from build123d import *

# Parameters (mm, degrees)
F0_W     = 44
F0_H     = 69
F1_DEPTH = 1200
F2_W     = 20
F2_H     = 44
F3_DEPTH = 44.001


with BuildPart() as f1:
    # F0 (on Top) → F1 (new body)
    with BuildSketch(Plane.XY):
        Rectangle(F0_W, F0_H)
    extrude(amount=F1_DEPTH)

    # F2 (on face) → F3 (cut, through all)
    with BuildSketch(Plane.YZ.offset(22)):
        Polygon((-0.5, 510), (34.5, 510), (34.5, 600), (34.5, 690), (-0.5, 690), (-0.5, 600), align=None)
        with Locations((24.5, 453)):
            Rectangle(F2_W, F2_H)
        with Locations((24.5, 747)):
            Rectangle(F2_W, F2_H)
    extrude(amount=-F3_DEPTH, mode=Mode.SUBTRACT)


solid = f1.part
Geometry check sheet. Reference: the model listing, model coordinates, mm. A direction names the side the tool comes from. Round coordinates to 2 decimals unless told otherwise and drop trailing zeros. Order: outer loops, then holes, each group sorted by start corner. A loop starts at its lowest first (then second) coordinate and runs counter-clockwise, first axis right, second up. Notation, with made-up numbers: M 86.5,70 L 125.5,70 A22 ccw 125.5,92 Z; hole C 37,7.5 d3. An arc over 180 degrees is marked long. Answer in a Markdown table with one row per item. Add a question column.
Item 1: Sectioned sample at A-A, the plane x = -10.5. Enter the section's corners in (y, z), plus the area to 3 significant figures.
Item 2: Sectioned sample at B-B, the plane z = 736.5. Enter the section's corners in (x, y), plus the area to 3 significant figures.
Item 3: Depth check by flat-ended pin: pin 1 Ø10 at (x, y) = (8.5, 24) entering from -Z; pin 2 Ø22 at (x, z) = (6, 609.5) entering from +Y. Enter the tip coordinate at first touch or a pass-through.
Item 4: Draft check along Z on faces 3 (the face through (0, 0, 1200)), 4 (the face through (0, 34.5, 981)), 5 (the face through (0, 0, 0)), 6 (the face through (0, 24, 725)). Enter one of: released by +Z, released by -Z, zero draft, split by the parting line, or undercut.
Item 5: Material ranges on L1, parallel to Z at x = 0, y = 23.5; L2, parallel to Y at x = -19, z = 670.5; L3, parallel to Y at x = 1, z = 434, recorded low to high. Write a range as [from, to].
Item 6: Set-up check for faces 1 (the face through (0, 14.5, 747)), 2 (the face through (-22, -8, 592)): record each of +Z, -Z, +X, -X, +Y, -Y from which the full face is reachable in a straight line by a thin tool's end or side.
Filled in:
| question | item | result |
|---|---|---|
| 1 | outline | M -34.5,0 L 34.5,0 L 34.5,431 L 14.5,431 L 14.5,475 L 34.5,475 L 34.5,510 L -0.5,510 L -0.5,690 L 34.5,690 L 34.5,725 L 14.5,725 L 14.5,769 L 34.5,769 L 34.5,1200 L -34.5,1200 Z |
| 1 | area | 74,700 mm² |
| 2 | outline | M -22,-34.5 L 22,-34.5 L 22,14.5 L -22,14.5 Z |
| 2 | area | 2,160 mm² |
| 3 | pin 1 | stops at z = 0 |
| 3 | pin 2 | stops at y = -0.5 |
| 4 | face 3 | released by +Z |
| 4 | face 4 | zero draft |
| 4 | face 5 | released by -Z |
| 4 | face 6 | undercut |
| 5 | L1 | z = [0, 431], [475, 510], [690, 725], [769, 1200] |
| 5 | L2 | y = [-34.5, -0.5] |
| 5 | L3 | y = [-34.5, 14.5] |
| 6 | face 1 | +X, -X, +Y |
| 6 | face 2 | +Z, -Z, -X, +Y, -Y |
